The listing builds one solid part. Answer for the finished solid, in the listing's coordinates (mm). Face numbers are marked on the shaded views. A direction names the side the tool comes from. Round coordinates to 2 decimals unless told otherwise and drop trailing zeros. Order: outer loops, then holes, each group sorted by start corner. A loop starts at its lowest first (then second) coordinate and runs counter-clockwise, first axis right, second up. Notation, with made-up numbers: (81.5, 82) -> (115.5, 82) arc R12 ccw to (115.5, 91) -> close; hole circle Ø9 at (-1, 30.5). An arc over 180 degrees is marked (long way). Return JSON: item names as keys, results as strings. Group by question number.
(1) The part is cut by section A-A (z = -2.5). Determine the outline of the cut face in (x, y), plus the area to 3 significant figures.
(2) The part is cut by section C-C (x = 12). Determine the outline of the cut face in (y, z).
(3) Which of the six approach directions +Z, -Z, +X, -X, +Y, -Y give full straight-line access (tool end or side, diameter ignored) to the marked faces 5 and 6?
(4) Consider line 1 (X direction, y = -16.25, z = -1); line 2 (Z direction, x = 79.5, y = -10). Determine where each line is inside the solid, lowest interval first. Write a range as [from, to].
(5) Determine the mould class of the marked faces 1, 2, 3 and 4 for opening direction X: +X half, -X half, draft (parallel to the pull), parting line (faces both ways), or undercut.
(6) The part is cut by section B-B (y = -10.25). Determine the outline of the cut face in (x, z), plus the area to 3 significant figures.
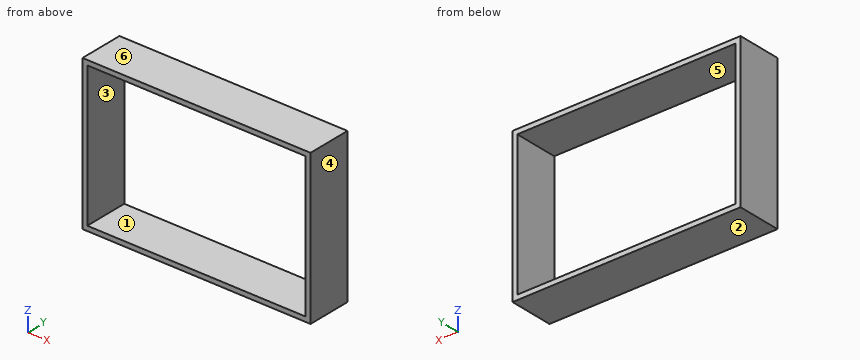
from build123d import *

# Parameters (mm, degrees)
SKETCH_2_W      = 2
SKETCH_2_H      = 10.4
SKETCH_2_H_2    = 18.3
SKETCH_2_H_3    = 13
EXTRUDE_1_DEPTH = 18.5


with BuildPart() as part:
    # 草图2 → 凸台-拉伸1 (new body)
    with BuildSketch(Plane(origin=(0, 0, 0), x_dir=(1, 0, 0), z_dir=(0, 1, 0))):
        Polygon((-0.2, 4.564103951), (-0.2, 5.3), (-2.2, 5.3), (-2.2, -2.2), (76.17, -2.2), (76.17, -0.2), (74.17, -0.2), (16.8, -0.2), (-0.2, -0.2), align=None)
        with Locations((-1.2, 10.5)):
            Rectangle(SKETCH_2_W, SKETCH_2_H)
        with Locations((-1.2, 24.85)):
            Rectangle(SKETCH_2_W, SKETCH_2_H_2)
        with Locations((-1.2, 40.5)):
            Rectangle(SKETCH_2_W, SKETCH_2_H_3)
        Polygon((-0.2, 50.2), (-0.2, 59.2), (13.8, 59.2), (16.8, 59.2), (74.17, 59.2), (76.17, 59.2), (91.37, 59.2), (91.37, -0.2), (76.17, -0.2), (76.17, -2.2), (93.37, -2.2), (93.37, 61.2), (-2.2, 61.2), (-2.2, 47), (-0.2, 47), align=None)
    extrude(amount=-EXTRUDE_1_DEPTH)


solid = part.part
Answer below:
{
 "1": {"outline": "(-2.2, -18.5) -> (-0.2, -18.5) -> (-0.2, 0) -> (-2.2, 0) -> close; (91.37, -18.5) -> (93.37, -18.5) -> (93.37, 0) -> (91.37, 0) -> close", "area": "74.0 mm²"},
 "2": {"outline": "(-18.5, -61.2) -> (0, -61.2) -> (0, -59.2) -> (-18.5, -59.2) -> close; (-18.5, 0.2) -> (0, 0.2) -> (0, 2.2) -> (-18.5, 2.2) -> close"},
 "3": {"face 5": "+Y, -Y", "face 6": "+Z, +X, -X, +Y, -Y"},
 "4": {"line 1": "x = [-2.2, -0.2], [91.37, 93.37]", "line 2": "z = [-61.2, -59.2], [0.2, 2.2]"},
 "5": {"face 1": "undercut", "face 2": "draft", "face 3": "undercut", "face 4": "+X half"},
 "6": {"outline": "(-2.2, -61.2) -> (93.37, -61.2) -> (93.37, 2.2) -> (-2.2, 2.2) -> close; hole (-0.2, -59.2) -> (91.37, -59.2) -> (91.37, 0.2) -> (-0.2, 0.2) -> close", "area": "620 mm²"}
}
